```python
from build123d import *

# Parameters (mm, degrees)
F0_R     = 7.5
F1_DEPTH = 205
F4_DEPTH = 10
F5_DEPTH = 15
F6_SIZE  = 0.5


with BuildPart() as f1:
    # F0 (on Top) → F1 (new body)
    with BuildSketch(Plane.XY):
        with Locations((-625.089943409, 134.0827345848)):
            Circle(F0_R)
    extrude(amount=F1_DEPTH)

    # F2 (on face) → F4 (cut)
    with BuildSketch(Plane.XY.offset(205)):
        with BuildLine():
            ThreePointArc((-617.589943409, 134.0827345848), (-618.81499321, 138.1906537661), (-622.089943409, 140.9565981272))
            Line((-622.089943409, 140.9565981272), (-622.089943409, 127.2088710424))
            ThreePointArc((-622.089943409, 127.2088710424), (-618.81499321, 129.9748154035), (-617.589943409, 134.0827345848))
        make_face()
    extrude(amount=-F4_DEPTH, mode=Mode.SUBTRACT)

    # F3 (on face) → F5 (cut)
    with BuildSketch(Plane(origin=(0, 0, 0), x_dir=(1, 0, 0), z_dir=(0, 0, -1))):
        with BuildLine():
            ThreePointArc((-617.589943409, -134.0827345848), (-618.81499321, -129.9748154035), (-622.089943409, -127.2088710424))
            Line((-622.089943409, -127.2088710424), (-622.089943409, -140.9565981272))
            ThreePointArc((-622.089943409, -140.9565981272), (-618.81499321, -138.1906537661), (-617.589943409, -134.0827345848))
        make_face()
    extrude(amount=-F5_DEPTH, mode=Mode.SUBTRACT)

    # F6
    f6_edges = [f1.edges().sort_by_distance(p)[0] for p in [
        (-632.589943, 134.082735, 0),
        (-632.589943, 134.082735, 205),
    ]]
    chamfer(f6_edges, length=F6_SIZE)


solid = f1.part
```
Geometry: final body of the model. Coordinates: model frame, mm. A direction names the side the tool comes from. Give positions to 0.01 mm unless a question says otherwise; leave off trailing zeros. Write each loop counter-clockwise with the first axis right and the second up, starting at its lowest first coordinate (ties: lowest second). Pieces come first, ordered by that corner, then holes.
1. Pin query (flat end, axial travel): P1, Ø2, axis at y = 138, z = 138, coming from the -X side; P2, Ø3, axis at x = -626, z = 134, coming from the +Y side; P3, Ø2, axis at y = 139, z = 104, coming from the -X side; P4, Ø4, axis at y = 131.5, z = 4.5, coming from the +X side. Return the tip coordinate at first contact, or that it passes through.
2. Line query: probe 1 along Z at (x, y) = (-621.5, 135); probe 2 along Y at (x, z) = (-624.5, 51); probe 3 along X at (y, z) = (134.25, 125). Output: solid intervals per line, ascending.
3. Reachability of faces 1 (the flat face through (-622.09, 134, 7)), 2 (the flat face through (-626, 134, 0)), 3 (the flat face through (-622.09, 134, 200)) from +Z, -Z, +X, -X, +Y, -Y: full face, straight path, thin tool, end or side. Return the list, or none.
4. Section query A-A, the plane z = 70.5. Return loops of the section in (x, y).
5. Section query B-B, the plane x = -619.25. Return loops of the section in (y, z), then the cut area to 3 significant figures.
Computed:
1. P1: stops at x = -632
1. P2: stops at y = 141.58
1. P3: stops at x = -631.49
1. P4: stops at x = -622.09
2. probe 1: z = 15 to 195
2. probe 2: y = 126.61 to 141.56
2. probe 3: x = -632.59 to -617.59
3. face 1: -Z, +X, +Y, -Y
3. face 2: -Z, +X, -X, +Y, -Y
3. face 3: +Z, +X, +Y, -Y
4. outline: circle Ø15 at (-625.09, 134.08)
5. outline: (129.38, 15) - (138.79, 15) - (138.79, 195) - (129.38, 195) - close
5. area: 1,690 mm2
